from build123d import *

# Parameters (mm, degrees)
BOSS_EXTRUDE1_DEPTH = 20
SKETCH2_R           = 15
CUT_EXTRUDE1_DEPTH  = 21
CHAMFER1_SIZE       = 2


with BuildPart() as part:
    # Sketch1 → Boss-Extrude1 (new body)
    with BuildSketch(Plane(origin=(0, 0, 0), x_dir=(1, 0, 0), z_dir=(0, 1, 0))):
        with BuildLine():
            Line((-80, 45), (80, 45))
            ThreePointArc((80, 45), (125, 0), (80, -45))
            Line((80, -45), (-80, -45))
            ThreePointArc((-80, -45), (-125, 0), (-80, 45))
        make_face()
    extrude(amount=BOSS_EXTRUDE1_DEPTH)

    # Sketch2 → Cut-Extrude1 (cut, through all)
    with BuildSketch(Plane(origin=(0, 20, 0), x_dir=(1, 0, 0), z_dir=(0, 1, 0))):
        with Locations((-80, 0)):
            Circle(SKETCH2_R)
        with Locations((80, 0)):
            Circle(SKETCH2_R)
    extrude(amount=-CUT_EXTRUDE1_DEPTH, mode=Mode.SUBTRACT)

    # Chamfer1
    chamfer1_edges = [part.edges().sort_by_distance(p)[0] for p in [
        (125, 20, 0),
        (0, 20, -45),
        (-125, 20, 0),
        (0, 0, -45),
        (125, 0, 0),
        (0, 0, 45),
        (-125, 0, 0),
        (0, 20, 45),
    ]]
    chamfer(chamfer1_edges, length=CHAMFER1_SIZE)


solid = part.part
Can you work these out from the model? Positions are in its coordinate system, mm. Give positions to 0.01 mm unless a question says otherwise; leave off trailing zeros. Loops run counter-clockwise (first coordinate to the right, second up) from the corner with the lowest first, then second, coordinate; pieces in that order, holes last. Notation, with made-up numbers: (75, 32.25) -> (122, 32.25) arc R18 cw to (122, 52.25) -> close; hole circle Ø5 at (62.5, -26.5). An arc over 180 degrees is marked (long way). Return JSON: item names as keys, results as strings.
Q1. I want a section at B-B, the plane y = 15. List the corners of the cut face in (x, z) for me, then the cut area to 3 significant figures.
Checks:
{"outline": "(-80, -45) -> (80, -45) arc R45 ccw to (80, 45) -> (-80, 45) arc R45 ccw to start; hole circle Ø30 at (-80, 0); hole circle Ø30 at (80, 0)", "area": "19,300 mm2"}
Q2. I need wall thicknesses on probe 1 along X at (y, z) = (10.75, 0); probe 2 along X at (y, z) = (18.5, 5.5); probe 3 along Z at (x, y) = (80, 10.5). Which ranges of each line are inside material? Lowest first, please.
Checks:
{"probe 1": "x = -125 to -95, -65 to 65, 95 to 125", "probe 2": "x = -124.16 to -93.96, -66.04 to 66.04, 93.96 to 124.16", "probe 3": "z = -45 to -15, 15 to 45"}
Q3. I want a section at C-C, the plane x = 74.5. List the corners of the cut face in (y, z) for me.
Checks:
{"outline": "(0, -43) -> (2, -45) -> (18, -45) -> (20, -43) -> (20, -13.96) -> (0, -13.96) -> close; (0, 13.96) -> (20, 13.96) -> (20, 43) -> (18, 45) -> (2, 45) -> (0, 43) -> close"}
Q4. For pin 1 Ø8 at (y, z) = (16, 9.5) entering from +X; pin 2 Ø8 at (y, z) = (7, -32.5) entering from -X; pin 3 Ø5 at (y, z) = (4.5, -27) entering from +X; pin 4 Ø18 at (x, z) = (80, 0) entering from +Y, each with a flat end and sliding along its axis, tell me the tip position at first contact or that it passes through.
Checks:
{"pin 1": "stops at x = 124.66", "pin 2": "stops at x = -114.82", "pin 3": "stops at x = 117.75", "pin 4": "passes through"}
Q5. I want a section at A-A, the plane z = 0. List the corners of the cut face in (x, y) for me, then the cut area to 3 significant figures.
Checks:
{"outline": "(-125, 2) -> (-123, 0) -> (-95, 0) -> (-95, 20) -> (-123, 20) -> (-125, 18) -> close; (-65, 0) -> (65, 0) -> (65, 20) -> (-65, 20) -> close; (95, 0) -> (123, 0) -> (125, 2) -> (125, 18) -> (123, 20) -> (95, 20) -> close", "area": "3,790 mm2"}
